Autodesk Inventor part; units mm, degrees
ref_plane "YZ Plane" through (0, 0, 0) normal (1, 0, 0) x (0, 1, 0)
ref_plane "XZ Plane" through (0, 0, 0) normal (0, 1, 0) x (-1, 0, 0)
ref_plane "XY Plane" through (0, 0, 0) normal (0, 0, 1) x (1, 0, 0)
sketch "Sketch1" plane through (0, 0, 0) normal (0, 0, 1) x (1, 0, 0)
  line L0 (0, 0) -> (560, 0)
  line L1 (560, 0) -> (560, 400)
  line L2 (560, 400) -> (0, 400)
  line L3 (0, 400) -> (0, 0)
  dimension "d0" = 560
  dimension "d1" = 400
extrude "Extrusion1" add sketch "Sketch1" along normal blind 8
sketch "Sketch2" plane through (0, 0, 8) normal (0, 0, 1) x (1, 0, 0)
  line L0 (181.25, 250) -> (378.75, 250)
  line L1 (378.75, 250) -> (378.75, 124)
  line L2 (378.75, 124) -> (181.25, 124)
  line L3 (181.25, 124) -> (181.25, 250)
  line L4 (0, 400) -> (0, 0)
  line L5 (560, 400) -> (0, 400)
  line L6 (186.25, 245) -> (373.75, 245)
  line L7 (373.75, 245) -> (373.75, 129)
  line L8 (373.75, 129) -> (186.25, 129)
  line L9 (186.25, 129) -> (186.25, 245)
  dimension "cuva_width" = 197.5
  dimension "d5" = 126
  dimension "d6" = 181.25
  dimension "d7" = 150
  dimension "d8" = 5
  dimension "d9" = 5
  dimension "d10" = 5
  dimension "d11" = 5
extrude "Extrusion2" cut sketch "Sketch2" against normal blind 4
fillet "Fillet1" radius 12 4 edges at (181.25, 250, 6) (181.25, 124, 6) (378.75, 124, 6) (378.75, 250, 6)
sketch "Sketch3" plane through (0, 0, 8) normal (0, 0, 1) x (1, 0, 0)
  line L0 (186.25, 245) -> (186.25, 129)
  line L1 (186.25, 129) -> (373.75, 129)
  line L2 (373.75, 129) -> (373.75, 245)
  line L3 (373.75, 245) -> (186.25, 245)
  point P0 (0, 0)
extrude "Extrusion3" cut sketch "Sketch3" against normal blind 4
sketch "Sketch4" plane through (0, 0, 4) normal (0, 0, 1) x (1, 0, 0)
  arc A0 (378.75, 238) -> (366.75, 250) centre (366.75, 238) ccw
  line L0 (193.25, 250) -> (366.75, 250)
  arc A1 (193.25, 250) -> (181.25, 238) centre (193.25, 238) ccw
  line L1 (181.25, 136) -> (181.25, 238)
  arc A2 (181.25, 136) -> (193.25, 124) centre (193.25, 136) ccw
  line L2 (366.75, 124) -> (193.25, 124)
  arc A3 (366.75, 124) -> (378.75, 136) centre (366.75, 136) ccw
  line L3 (378.75, 238) -> (378.75, 136)
  line L4 (198.25, 245) -> (361.75, 245)
  line L5 (373.75, 233) -> (373.75, 141)
  line L6 (361.75, 129) -> (198.25, 129)
  line L7 (186.25, 141) -> (186.25, 233)
  arc A4 (198.25, 245) -> (186.25, 233) centre (198.25, 233) ccw
  arc A5 (186.25, 141) -> (198.25, 129) centre (198.25, 141) ccw
  arc A6 (373.75, 233) -> (361.75, 245) centre (361.75, 233) ccw
  arc A7 (361.75, 129) -> (373.75, 141) centre (361.75, 141) ccw
  point P0 (0, 0)
  dimension "d17" = 5
  dimension "d18" = 5
  dimension "d19" = 5
  dimension "d20" = 5
  dimension "d21" = 12
extrude "Extrusion4" cut sketch "Sketch4" against normal through all contours L4 A6 L5 A7 L6 A5 L7 A4
equation "\"d9\" = d8"
equation "\"d10\" = d8"
equation "\"d11\" = d8"
equation "\"d18\" = d17"
equation "\"d19\" = d17"
equation "\"d20\" = d17"
properties part number "capac cu gaura 3"
Part model, mm, in its own coordinate system. A direction names the side the tool comes from. Round coordinates to 2 decimals unless told otherwise and drop trailing zeros. Loops run counter-clockwise (first coordinate to the right, second up) from the corner with the lowest first, then second, coordinate; pieces in that order, holes last. Notation, with made-up numbers: (62, -1) - (104, -1) arc R10 ccw to (104, 13) - close; hole circle Ø9 at (50.25, 49.25). An arc over 180 degrees is marked (long way). Answer as a JSON object with one key per item and string values.
Item 1: Band-saw the part on C-C on z = 2. List the corners of the cut face in (x, y).
Output:
{"outline": "(0, 0) - (560, 0) - (560, 400) - (0, 400) - close; hole (186.25, 141) arc R12 ccw to (198.25, 129) - (361.75, 129) arc R12 ccw to (373.75, 141) - (373.75, 233) arc R12 ccw to (361.75, 245) - (198.25, 245) arc R12 ccw to (186.25, 233) - close"}
Item 2: Wall check: L1, parallel to Y at x = 251, z = 5.75; L2, parallel to X at y = 204.5, z = 6.25; L3, parallel to Y at x = 313.5, z = 3. Give the ranges that are in metal, low to high.
Output:
{"L1": "0 to 124, 250 to 400", "L2": "0 to 181.25, 378.75 to 560", "L3": "0 to 129, 245 to 400"}
Item 3: Band-saw the part on B-B on y = 226. List the corners of the cut face in (x, z), plus the area to 3 significant figures.
Output:
{"outline": "(0, 0) - (186.25, 0) - (186.25, 4) - (181.25, 4) - (181.25, 8) - (0, 8) - close; (373.75, 0) - (560, 0) - (560, 8) - (378.75, 8) - (378.75, 4) - (373.75, 4) - close", "area": "2,940 mm2"}
Item 4: Tool access for faces 3 (the face through (276, 247, 0)), 4 (the face through (189.86, 241.58, 2.03)), 5 (the face through (280, 248, 4)): list every direction of +Z, -Z, +X, -X, +Y, -Y with a clear straight run to the whole face (end or side of a thin tool).
Output:
{"face 3": "-Z, +X, -X, +Y, -Y", "face 4": "+Z, -Z", "face 5": "+Z"}
Item 5: Band-saw the part on A-A on x = 257.5. List the corners of the cut face in (y, z).
Output:
{"outline": "(0, 0) - (129, 0) - (129, 4) - (124, 4) - (124, 8) - (0, 8) - close; (245, 0) - (400, 0) - (400, 8) - (250, 8) - (250, 4) - (245, 4) - close"}
Item 6: Pull direction X, two halves, no side cores. Call faces 1 (the face through (276, 292, 8)), 2 (the face through (189.67, 132.61, 2.03)): pulls with the +X half, pulls with the -X half, needs draft (parallel to the pull), parting line crosses it, or undercut.
Output:
{"face 1": "needs draft", "face 2": "undercut"}
